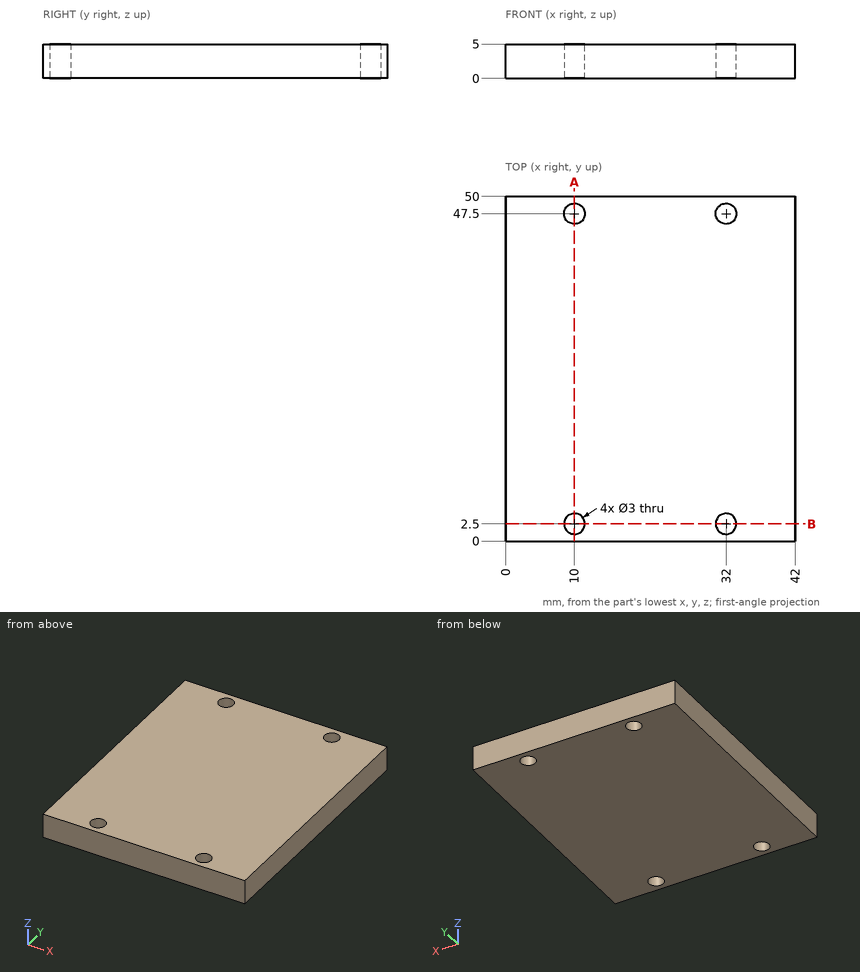
Geometry: see drawing. Coordinates: mm, zero at the bounding-box minimum. Give positions to 0.01 mm unless a question says otherwise; leave off trailing zeros. Order: outer loops, then holes, each group sorted by start corner. A loop starts at its lowest first (then second) coordinate and runs counter-clockwise, first axis right, second up. Notation, with made-up numbers: M 26,66 L 68,66 A27 ccw 68,96 Z; hole C -23.5,43.5 d5. An arc over 180 degrees is marked long. Answer as CSV lines item,"result". Start each with the question number.
1) Line query: line 1 (Y direction, x = 10, z = 1.2); line 2 (X direction, y = 47.5, z = 3.05); line 3 (Y direction, x = 31, z = 0.75). Output: solid intervals per line, ascending. Write a range as from..to.
2) Cut plane B-B (y = 2.5). Output: boundary loops of the cut face in (x, z).
3) Cut plane A-A (x = 10). Output: boundary loops of the cut face in (y, z), then the cut area to 3 significant figures.
4) First-contact query: P1, Ø2, axis at x = 31.5, y = 21, coming from the -Z side; P2, Ø2.5, axis at x = 32, y = 47.5, coming from the -Z side. Flat tips, straight axial feed; report the tip coordinate or a pass-through.
Findings below:
1,line 1,"y = 0..1, 4..46, 49..50"
1,line 2,"x = 0..8.5, 11.5..30.5, 33.5..42"
1,line 3,"y = 0..1.38, 3.62..46.38, 48.62..50"
2,outline,"M 0,0 L 8.5,0 L 8.5,5 L 0,5 Z; M 11.5,0 L 30.5,0 L 30.5,5 L 11.5,5 Z; M 33.5,0 L 42,0 L 42,5 L 33.5,5 Z"
3,outline,"M 0,0 L 1,0 L 1,5 L 0,5 Z; M 4,0 L 46,0 L 46,5 L 4,5 Z; M 49,0 L 50,0 L 50,5 L 49,5 Z"
3,area,"220 mm²"
4,P1,"stops at z = 0"
4,P2,"passes through"
